Read the model definition and answer for the solid it produces. Units are mm, in the model's axes. A direction names the side the tool comes from. Give positions to 0.01 mm unless a question says otherwise; leave off trailing zeros. Order: outer loops, then holes, each group sorted by start corner. A loop starts at its lowest first (then second) coordinate and runs counter-clockwise, first axis right, second up.
```python
from build123d import *

# Parameters (mm, degrees)
SKETCH1_R           = 19.05
SKETCH1_R_2         = 12.827
BASE_EXTRUDE_DEPTH  = 127
SKETCH2_W           = 9.525
SKETCH2_H           = 25.4
BOSS_EXTRUDE1_DEPTH = 57.754917
SKETCH3_R           = 4.064
CUT_EXTRUDE1_DEPTH  = 24.8125
CIRPATTERN1_COUNT   = 3
SKETCH6_R           = 4.064
CUT_EXTRUDE2_DEPTH  = 76.516135768
SKETCH7_R           = 4.064
CUT_EXTRUDE3_DEPTH  = 76.516135768
SKETCH10_R          = 7.1501
CUT_EXTRUDE4_DEPTH  = 0.635
SKETCH13_W          = 12.7
SKETCH13_H          = 25.4
BOSS_EXTRUDE3_DEPTH = 39.189488
CIRPATTERN2_COUNT   = 3
FILLET1_R           = 3.175
FILLET2_R           = 3.175
FILLET3_R           = 3.175


with BuildPart() as part:
    # Sketch1 → Base-Extrude (new body)
    with BuildSketch(Plane.XY):
        Circle(SKETCH1_R)
        Circle(SKETCH1_R_2, mode=Mode.SUBTRACT)
    extrude(amount=BASE_EXTRUDE_DEPTH)

    # Sketch2 → Boss-Extrude1 (add)
    with BuildSketch(Plane(origin=(0, -76.2, 0), x_dir=(-1, 0, 0), z_dir=(0, 1, 0))):
        with Locations((0, 12.7)):
            Rectangle(SKETCH2_W, SKETCH2_H)
    boss_extrude1 = extrude(amount=BOSS_EXTRUDE1_DEPTH)

    # Sketch3 → Cut-Extrude1 (cut, through all)
    with BuildSketch(Plane.ZY.offset(4.7625)):
        with Locations((9.525, -66.675)):
            Circle(SKETCH3_R)
    extrude(amount=-CUT_EXTRUDE1_DEPTH, mode=Mode.SUBTRACT)

    # CirPattern1: Boss-Extrude1 ×3 about axis
    cirpattern1_axis = Axis((0, 0, 0), (0, 0, 1))
    for i in range(1, CIRPATTERN1_COUNT):
        add(boss_extrude1.rotate(cirpattern1_axis, i * 360 / CIRPATTERN1_COUNT))

    # Sketch6 → Cut-Extrude2 (cut, through all)
    with BuildSketch(Plane(origin=(-45.618861607, 20.838800715, 50.936831184), x_dir=(0.866025404, -0.5, 0), z_dir=(-0.5, -0.866025404, 0))):
        with Locations((-16.748506599, -41.411831184)):
            Circle(SKETCH6_R)
    extrude(amount=-CUT_EXTRUDE2_DEPTH, mode=Mode.SUBTRACT)

    # Sketch7 → Cut-Extrude3 (cut, through all)
    with BuildSketch(Plane(origin=(34.377585278, 14.3486468, 49.693003082), x_dir=(0.866025404, 0.5, 0), z_dir=(0.5, -0.866025404, 0))):
        with Locations((29.728814428, -40.168003082)):
            Circle(SKETCH7_R)
    extrude(amount=-CUT_EXTRUDE3_DEPTH, mode=Mode.SUBTRACT)

    # Sketch10 → Cut-Extrude4 (cut)
    with BuildSketch(Plane(origin=(0, 15.875, 0), x_dir=(-1, 0, 0), z_dir=(0, 1, 0))):
        with Locations((0, 38.1)):
            Circle(SKETCH10_R)
    extrude(amount=-CUT_EXTRUDE4_DEPTH, mode=Mode.SUBTRACT)

    # Sketch12 → Hole2 (revolve, cut)
    with BuildSketch(Plane(origin=(0, 15.24, 38.1), x_dir=(0, 0, 1), z_dir=(1, 0, 0))):
        Polygon((0, 0), (0, 14.233804302), (2.552697789, 12.699989), (2.552697789, 9.52499175), (3.17499725, 9.52499175), (3.17499725, 0.002539998), (3.17499725, 0), align=None)
    revolve(axis=Axis((0, 15.24, 38.1), (0, -1, 0)), mode=Mode.SUBTRACT)

    # Sketch13 → Boss-Extrude3 (add)
    with BuildSketch(Plane(origin=(0, -57.15, 0), x_dir=(-1, 0, 0), z_dir=(0, 1, 0))):
        with Locations((0, 12.7)):
            Rectangle(SKETCH13_W, SKETCH13_H)
    boss_extrude3 = extrude(amount=BOSS_EXTRUDE3_DEPTH)

    # CirPattern2: Boss-Extrude3 ×3 about axis
    cirpattern2_axis = Axis((0, 0, 0), (0, 0, 1))
    for i in range(1, CIRPATTERN2_COUNT):
        add(boss_extrude3.rotate(cirpattern2_axis, i * 360 / CIRPATTERN2_COUNT))

    # Fillet1
    fillet1_edges = [part.edges().sort_by_distance(p)[0] for p in [
        (-12.379259657, 14.479517314, 12.7),
        (12.379259657, 14.479517314, 12.7),
    ]]
    fillet(fillet1_edges, radius=FILLET1_R)

    # Fillet2
    fillet2_edges = [part.edges().sort_by_distance(p)[0] for p in [
        (-18.729259657, 3.480994686, 12.7),
        (-6.35, -17.960512, 12.7),
    ]]
    fillet(fillet2_edges, radius=FILLET2_R)

    # Fillet3
    fillet3_edges = [part.edges().sort_by_distance(p)[0] for p in [
        (18.729259657, 3.480994686, 12.7),
        (6.35, -17.960512, 12.7),
    ]]
    fillet(fillet3_edges, radius=FILLET3_R)


solid = part.part
```
1) Given pin 1 (13 mm diameter, centred on x = 3, y = -40.5, fed in from +Z); pin 2 (0.8 mm diameter, centred on x = 5.5, z = 8, fed in from -Y); pin 3 (2 mm diameter, centred on y = 30, z = 16, fed in from +X), each flat-ended and moving along its own axis, determine where each tip first touches the part or whether it passes through.
Final values:
pin 1: stops at z = 25.4
pin 2: stops at y = -57.15
pin 3: stops at x = 63.22
2) The part is cut by section C-C on y = -37. Determine the outline of the cut face in (x, z).
Final values:
outline: (-6.35, 0) - (6.35, 0) - (6.35, 25.4) - (-6.35, 25.4) - close
3) Consider L1, parallel to Y at x = 0, z = 32 (3 decimals); L2, parallel to Z at x = 0, y = 13 (3 decimals); L3, parallel to Y at x = 0, z = 96. Determine where each line is inside the solid, lowest interval first.
Final values:
L1: y = -19.05 to -12.827, 12.827 to 15.24, 15.875 to 19.05
L2: z = 0 to 34.925, 41.275 to 127
L3: y = -19.05 to -12.83, 12.83 to 19.05
4) The part is cut by section D-D on z = 99. Determine the outline of the cut face in (x, y).
Final values:
outline: circle Ø38.1 at (0, 0); hole circle Ø25.65 at (0, 0)
5) For a pull along Z with two mould halves and no side action, classify faces 1 (the face through (41, 24, 25.4)), 2 (the face through (-54.42, 31.34, 10.75)), 3 (the face through (-3.84, 15.56, 44.13)), 4 (the face through (-4.762, -67, 15)) as released by +Z, released by -Z, zero draft, split by the parting line, or undercut.
Final values:
face 1: released by +Z
face 2: undercut
face 3: undercut
face 4: zero draft
6) The part is cut by section A-A on z = 38.1. Determine the outline of the cut face in (x, y) (3 decimals).
Final values:
outline: circle Ø38.1 at (0, 0); hole (-7.15, 15.24) - (-3.175, 15.24) - (-3.175, 12.428) arc R12.827 ccw (long way) to (3.175, 12.428) - (3.175, 15.24) - (7.15, 15.24) - (7.15, 15.875) - (-7.15, 15.875) - close
7) A tool of negligible diameter and unlimited length cuts with its end or side. For faces 5 (the face through (-66.024, 38.042, 12.878)), 6 (the face through (-6.35, -39, 13)), 7 (the face through (1.22, 13.81, 41.03)), 8 (the face through (6.35, -39, 13)), 9 (the face through (-30.491, 24.937, 12.522)), from which of +Z, -Z, +X, -X, +Y, -Y can it reach the whole face along a straight path? Write none if from no direction.
Final values:
face 5: +Z, -Z, -X, +Y
face 6: +Z, -Z, -X, -Y
face 7: none
face 8: +Z, -Z, +X, -Y
face 9: +Z, -Z, +Y
8) The part is cut by section B-B on x = 0. Determine the outline of the cut face in (y, z) (3 decimals).
Final values:
outline: (-76.2, 0) - (-12.827, 0) - (-12.827, 127) - (-19.05, 127) - (-19.05, 25.4) - (-76.2, 25.4) - close; (12.827, 0) - (19.05, 0) - (19.05, 127) - (12.827, 127) - (12.827, 41.275) - (15.24, 41.275) - (15.24, 45.25) - (15.875, 45.25) - (15.875, 30.95) - (15.24, 30.95) - (15.24, 34.925) - (12.827, 34.925) - close; hole circle Ø8.128 at (-66.675, 9.525)
